The model under review builds one solid part; all positions refer to its coordinate system, in mm. Round coordinates to 2 decimals unless told otherwise and drop trailing zeros. Loops run counter-clockwise (first coordinate to the right, second up) from the corner with the lowest first, then second, coordinate; pieces in that order, holes last. Notation, with made-up numbers: M 57.25,42.25 L 72.25,42.25 A13 cw 72.25,58.25 Z; hole C -39,62 d2. An arc over 180 degrees is marked long. Answer as a JSON object with one key per item and string values. Group by question number.
Item 1: Consider section B-B (y = -119.5). Give the boundary of the cut face in (x, z).
Item 2: Insertion check: P1, Ø3.5, axis at x = 0, y = 0, coming from the -Z side. The pin has a flat end and moves straight along its axis. Give the tip position at first contact, or say it passes through.
Item 3: Consider section C-C (x = -78.5). Give the boundary of the cut face in (y, z).
Item 4: To check wall thickness, follow line 1 (Y direction, x = 0, z = 0.15); line 2 (X direction, y = -90, z = -0.35); line 3 (X direction, y = 0, z = -0.35). State the ranges of each line that lie inside material, in increasing order.
Item 5: Consider section A-A (z = -0.85). Give the boundary of the cut face in (x, y), and give its area (3 significant figures).
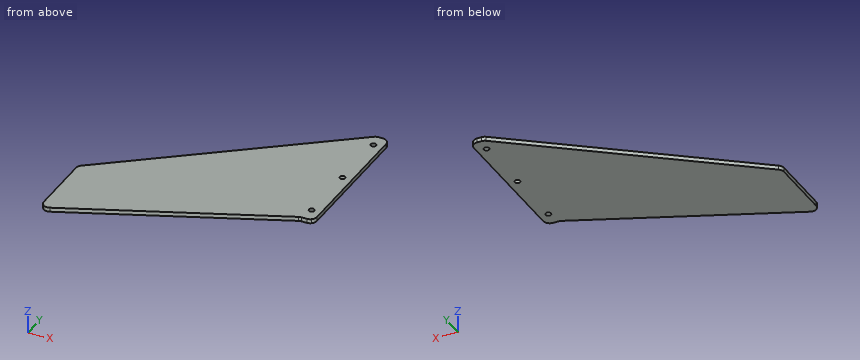
```python
from build123d import *

# Parameters (mm, degrees)
EXTRUDE_1_DEPTH      = 1.6
EXTRUDE_1_DEPTH_BACK = 1.6


with BuildPart() as part:
    # Эскиз1 → Бобышка-Вытянуть1 (new, two sides: drawn at the far end of the back side and taken through both)
    with BuildSketch(Plane.XY.offset(-EXTRUDE_1_DEPTH_BACK)):
        with BuildLine():
            Line((-4.348647769, 8.961289917), (-162.050931365, -112.49885397))
            ThreePointArc((-162.050931365, -112.49885397), (-163.486349118, -114.252731015), (-164, -116.460143887))
            Line((-164, -116.460143887), (-164, -163.373940781))
            ThreePointArc((-164, -163.373940781), (-161.741518486, -167.555337245), (-157.006369443, -167.959291062))
            Line((-157.006369443, -167.959291062), (-3.953694353, -101.414649719))
            ThreePointArc((-3.953694353, -101.414649719), (-2.978211279, -101.104759893), (-1.960063796, -101))
            Line((-1.960063796, -101), (2, -101))
            ThreePointArc((2, -101), (3.586523282, -100.741618276), (5.009075116, -99.99317755))
            ThreePointArc((5.009075116, -99.99317755), (6.474671808, -98.230989066), (7, -96))
            Line((7, -96), (7, 5))
            ThreePointArc((7, 5), (5.535533906, 8.535533906), (2, 10))
            Line((2, 10), (-1.297716404, 10))
            ThreePointArc((-1.297716404, 10), (-2.909167678, 9.733204495), (-4.348647769, 8.961289917))
        make_face()
        with BuildLine():
            ThreePointArc((1.203630046, -1.59727102), (1.59727102, 1.203630046), (-1.203630046, 1.59727102))
            ThreePointArc((-1.203630046, 1.59727102), (-1.59727102, -1.203630046), (1.203630046, -1.59727102))
        make_face(mode=Mode.SUBTRACT)
        with BuildLine():
            ThreePointArc((1.203630046, -46.59727102), (1.59727102, -43.796369954), (-1.203630046, -43.40272898))
            ThreePointArc((-1.203630046, -43.40272898), (-1.59727102, -46.203630046), (1.203630046, -46.59727102))
        make_face(mode=Mode.SUBTRACT)
        with BuildLine():
            ThreePointArc((1.203630046, -91.59727102), (1.59727102, -88.796369954), (-1.203630046, -88.40272898))
            ThreePointArc((-1.203630046, -88.40272898), (-1.59727102, -91.203630046), (1.203630046, -91.59727102))
        make_face(mode=Mode.SUBTRACT)
    extrude(amount=EXTRUDE_1_DEPTH + EXTRUDE_1_DEPTH_BACK)


solid = part.part
```
Geometry results:
{
 "1": {"outline": "M -164,-1.6 L -45.55,-1.6 L -45.55,1.6 L -164,1.6 Z"},
 "2": {"P1": "passes through"},
 "3": {"outline": "M -133.83,-1.6 L -48.15,-1.6 L -48.15,1.6 L -133.83,1.6 Z"},
 "4": {"line 1": "y = -101 to -92, -88 to -47, -43 to -2, 2 to 10", "line 2": "x = -132.84 to -2, 2 to 7", "line 3": "x = -15.98 to -2, 2 to 7"},
 "5": {"outline": "M -164,-163.37 A5 ccw -157.01,-167.96 L -3.95,-101.41 A5 cw -1.96,-101 L 2,-101 A5 ccw 7,-96 L 7,5 A5 ccw 2,10 L -1.3,10 A5 ccw -4.35,8.96 L -162.05,-112.5 A5 ccw -164,-116.46 Z; hole C 0,-90 d4; hole C 0,-45 d4; hole C 0,0 d4", "area": "14,600 mm^2"}
}
